```python
from build123d import *

# Parameters (mm, degrees)
F1_DEPTH = 50.8
F2_D     = 15.875
F2_DEPTH = 15.875
F2_TIP   = 4.7693311635
F4_D     = 15.875
F4_DEPTH = 15.875
F4_TIP   = 4.7693311635


with BuildPart() as f1:
    # F0 (on Top) → F1 (new body)
    with BuildSketch(Plane.XY):
        Polygon((6.4158048664, 11.1125), (-6.4158048664, 11.1125), (-12.8316097327, 0), (-6.4158048664, -11.1125), (6.4158048664, -11.1125), (12.8316097327, 0), align=None)
    extrude(amount=F1_DEPTH)

    # F2
    with Locations(Plane(origin=(0, 0, 0), x_dir=(1, 0, 0), z_dir=(0, 0, -1))):
        with Locations((0, 0)):
            Hole(F2_D / 2, depth=F2_DEPTH)
            with Locations((0, 0, -(F2_DEPTH + F2_TIP / 2))):  # 118° drill point
                Cone(0, F2_D / 2, F2_TIP, mode=Mode.SUBTRACT)

    # F4
    with Locations(Plane.XY.offset(50.8)):
        with Locations((0, 0)):
            Hole(F4_D / 2, depth=F4_DEPTH)
            with Locations((0, 0, -(F4_DEPTH + F4_TIP / 2))):  # 118° drill point
                Cone(0, F4_D / 2, F4_TIP, mode=Mode.SUBTRACT)


solid = f1.part
```
Geometry: final body of the model. Coordinates: model frame, mm. A direction names the side the tool comes from. Give positions to 0.01 mm unless a question says otherwise; leave off trailing zeros. Loops run counter-clockwise (first coordinate to the right, second up) from the corner with the lowest first, then second, coordinate; pieces in that order, holes last. Notation, with made-up numbers: (44.25, -19.75) -> (92.25, -19.75) arc R5 cw to (92.25, -11.75) -> close; hole circle Ø1 at (49.5, 60). An arc over 180 degrees is marked (long way). Use CSV: the item, a comma, the result in double quotes.
(1) Pull-direction query (Y, two-part tool) for faces 4 (the face through (3, 8, 0)), 5 (the face through (-1.016, 0.932, 30.984)), 6 (the face through (9.67, 5.48, 25.04)); classes: released by +Y, released by -Y, zero draft, split by the parting line, or undercut.
From the geometry:
face 4,"zero draft"
face 5,"undercut"
face 6,"released by +Y"
(2) Cut plane B-B (y = 8.75). Output: boundary loops of the cut face in (x, z), plus the area to 3 significant figures.
From the geometry:
outline,"(-7.78, 0) -> (7.78, 0) -> (7.78, 50.8) -> (-7.78, 50.8) -> close"
area,"790 mm^2"
(3) Access query for faces 1 (the face through (0, -11.112, 25)), 2 (the face through (1.72, -7.75, 42.75)), 3 (the face through (1.72, 7.75, 8.05)). Directions: +Z, -Z, +X, -X, +Y, -Y. A direction counts if a zero-diameter tool reaches every point of the face in a straight line with its end or side. Return the directions, or none.
From the geometry:
face 1,"+Z, -Z, +X, -X, -Y"
face 2,"+Z"
face 3,"-Z"
(4) Ray query, line 1 along Y through (x, z) = (0, 12.25); line 2 along X through (y, z) = (0, 44); line 3 along Y through (x, z) = (-8.25, 47). Return the intervals inside material, ascending. Write a range as [from, to].
From the geometry:
line 1,"[-11.11, -7.94], [7.94, 11.11]"
line 2,"[-12.83, -7.94], [7.94, 12.83]"
line 3,"[-7.94, 7.94]"
(5) Cut plane A-A (z = 15). Output: boundary loops of the cut face in (x, y) (1 decimal), plus the area to 3 significant figures.
From the geometry:
outline,"(-12.8, 0) -> (-6.4, -11.1) -> (6.4, -11.1) -> (12.8, 0) -> (6.4, 11.1) -> (-6.4, 11.1) -> close; hole circle Ø15.9 at (0, 0)"
area,"230 mm^2"
(6) First-contact query: P1, Ø2, axis at x = -10, z = 22.5, coming from the +Y side; P2, Ø9.5, axis at x = 0, y = 0, coming from the -Z side; P3, Ø2, axis at y = -8, z = 11, coming from the -X side. Flat tips, straight axial feed; report the tip coordinate or a pass-through.
From the geometry:
P1,"y = 6.64"
P2,"z = 17.79"
P3,"x = -8.79"
